```python
from build123d import *

# Parameters (mm, degrees)
F1_DEPTH = 15


with BuildPart() as f1:
    # F0 (on Front) → F1 (new body)
    with BuildSketch(Plane.XZ):
        with BuildLine():
            ThreePointArc((-44.369697, 3), (-43.491018, 0.87868), (-41.369697, 0))
            Line((-41.369697, 0), (-34.154815, 0))
            ThreePointArc((-34.154815, 0), (-27.654815, -6.5), (-21.154815, 0))
            Line((-21.154815, 0), (4.982472, 0))
            ThreePointArc((4.982472, 0), (11.482472, -6.5), (17.982472, 0))
            Line((17.982472, 0), (24.432209, 0))
            ThreePointArc((24.432209, 0), (26.553529, 0.87868), (27.432209, 3))
            Line((27.432209, 3), (27.432209, 3.964023))
            ThreePointArc((27.432209, 3.964023), (26.553529, 6.085343), (24.432209, 6.964023))
            Line((24.432209, 6.964023), (24.333949, 6.964023))
            Line((24.333949, 6.964023), (24.333949, 10.970772))
            ThreePointArc((24.333949, 10.970772), (21.990804, 16.627626), (16.333949, 18.970772))
            Line((16.333949, 18.970772), (10.616395, 18.970772))
            Line((10.616395, 18.970772), (10.616395, 25.112818))
            ThreePointArc((10.616395, 25.112818), (10.030609, 26.527032), (8.616395, 27.112818))
            Line((8.616395, 27.112818), (-16.014689, 27.112818))
            ThreePointArc((-16.014689, 27.112818), (-21.671543, 24.769673), (-24.014689, 19.112818))
            Line((-24.014689, 19.112818), (-24.014689, 18.970772))
            Line((-24.014689, 18.970772), (-29.21758, 18.970772))
            ThreePointArc((-29.21758, 18.970772), (-37.702862, 15.456053), (-41.21758, 6.970772))
            Line((-41.21758, 6.970772), (-41.21758, 6.964023))
            Line((-41.21758, 6.964023), (-41.369697, 6.964023))
            ThreePointArc((-41.369697, 6.964023), (-43.491018, 6.085343), (-44.369697, 3.964023))
            Line((-44.369697, 3.964023), (-44.369697, 3))
        make_face()
        with BuildLine():
            ThreePointArc((-19.692936, 22.499631), (-18.022914, 23.691795), (-16.014689, 24.112818))
            Line((-16.014689, 24.112818), (5.616395, 24.112818))
            ThreePointArc((5.616395, 24.112818), (7.030609, 23.527032), (7.616395, 22.112818))
            Line((7.616395, 22.112818), (7.616395, 21.144906))
            ThreePointArc((7.616395, 21.144906), (7.030609, 19.730692), (5.616395, 19.144906))
            Line((5.616395, 19.144906), (-18.221637, 19.144906))
            ThreePointArc((-18.221637, 19.144906), (-20.053228, 20.341616), (-19.692936, 22.499631))
        make_face(mode=Mode.SUBTRACT)
    extrude(amount=F1_DEPTH)


solid = f1.part
```
Input: part model. Units: mm. Frame: model coordinates. A direction names the side the tool comes from. Round coordinates to 2 decimals unless told otherwise and drop trailing zeros. Loops run counter-clockwise (first coordinate to the right, second up) from the corner with the lowest first, then second, coordinate; pieces in that order, holes last. Notation, with made-up numbers: (5.25, 71.5) -> (36.25, 71.5) arc R24 cw to (36.25, 86.5) -> close; hole circle Ø1 at (-15.75, -1). An arc over 180 degrees is marked (long way). Use one line per item in the form item = value. Start each with the question number.
Item 1: Material intervals for L1, parallel to Z at x = -4.5, y = -2.5; L2, parallel to X at y = -13.5, z = -4; L3, parallel to X at y = -6, z = -3, sorted ascending. Write a range as from..to.
Item 2: Section query C-C on x = 12.5. Return the cut outline in (y, z).
Item 3: Contact query for flat-ended pins moving along their axis: pin 1 Ø8 at (x, z) = (-22, 0) entering from +Y; pin 2 Ø1.9 at (x, y) = (22, -7) entering from -Z; pin 3 Ø3 at (x, y) = (13, -4.5) entering from +Z; pin 4 Ø2 at (x, y) = (-32.5, -7) entering from -Z. Output: stop coordinate, or through.
Item 4: Section query A-A on x = -13. Return the cut outline in (y, z), then the cut area to 3 significant figures.
Item 5: Set-up query: faces 5 (the face through (7.015, -7.395, 23.542)), 6 (the face through (21, -7, 0)), 7 (the face through (10.616, -7, 22)), 8 (the face through (-8, -7, 0)). Return all of +Z, -Z, +X, -X, +Y, -Y with unobstructed straight access to the full face (end or side cutting, diameter ignored); none if empty.
Item 6: Mould query, pull axis X, two halves, no side actions, for faces 1 (the face through (-38, -7, 0)), 2 (the face through (-20.04, -7.4, 20.31)), 3 (the face through (-6, -7, 19.145)), 4 (the face through (26.58, -7.4, 6.06)). Classes: pulls with the +X half, pulls with the -X half, needs draft (parallel to the pull), parting line crosses it, or undercut.
Item 7: Section query D-D on z = 10. Return the cut outline in (x, y).
Ans:
q1.L1 = 0..19.14, 24.11..27.11
q1.L2 = -32.78..-22.53, 6.36..16.61
q1.L3 = -33.42..-21.89, 5.72..17.25
q2.outline = (-15, -6.42) -> (0, -6.42) -> (0, 18.97) -> (-15, 18.97) -> close
q3.pin_1 = 0
q3.pin_2 = 0
q3.pin_3 = 18.97
q3.pin_4 = -5.24
q4.outline = (-15, 0) -> (0, 0) -> (0, 19.14) -> (-15, 19.14) -> close; (-15, 24.11) -> (0, 24.11) -> (0, 27.11) -> (-15, 27.11) -> close
q4.area = 332 mm^2
q5.face_5 = +Y, -Y
q5.face_6 = -Z, +X, +Y, -Y
q5.face_7 = +Z, +X, +Y, -Y
q5.face_8 = -Z, +Y, -Y
q6.face_1 = needs draft
q6.face_2 = undercut
q6.face_3 = undercut
q6.face_4 = pulls with the +X half
q7.outline = (-40.83, -15) -> (24.33, -15) -> (24.33, 0) -> (-40.83, 0) -> close
